```python
from build123d import *

# Parameters (mm, degrees)
MODEL_R             = 1.75
MODEL_R_2           = 2.25
MODEL_R_3           = 15
MODEL_R_4           = 2.75
MODEL_R_5           = 10.5
MODEL_R_6           = 4.25
BOSS_EXTRUDE1_DEPTH = 18


with BuildPart() as part:
    # Model → Boss-Extrude1 (new body)
    with BuildSketch(Plane.XY):
        Polygon((195, 0), (205, 10), (205, 141.83), (195, 151.83), (160.9225, 151.83), (95.411764706, 258.588235294), (54, 300), (16, 300), (0, 284), (0, 90), (10, 80), (65, 80), (75, 70), (75, 10), (85, 0), align=None)
        with Locations((60, 279.7)):
            Circle(MODEL_R, mode=Mode.SUBTRACT)
        with Locations((10, 279.7)):
            Circle(MODEL_R, mode=Mode.SUBTRACT)
        with Locations((10, 224.7)):
            Circle(MODEL_R, mode=Mode.SUBTRACT)
        with Locations((10, 154.7)):
            Circle(MODEL_R, mode=Mode.SUBTRACT)
        with Locations((10, 99.7)):
            Circle(MODEL_R, mode=Mode.SUBTRACT)
        with Locations((60, 99.7)):
            Circle(MODEL_R, mode=Mode.SUBTRACT)
        with Locations((60, 154.7)):
            Circle(MODEL_R, mode=Mode.SUBTRACT)
        with Locations((60, 224.7)):
            Circle(MODEL_R, mode=Mode.SUBTRACT)
        with Locations((10, 252.2)):
            Circle(MODEL_R, mode=Mode.SUBTRACT)
        with Locations((60, 252.2)):
            Circle(MODEL_R, mode=Mode.SUBTRACT)
        with Locations((35, 224.7)):
            Circle(MODEL_R, mode=Mode.SUBTRACT)
        with Locations((10, 189.7)):
            Circle(MODEL_R, mode=Mode.SUBTRACT)
        with Locations((60, 189.7)):
            Circle(MODEL_R, mode=Mode.SUBTRACT)
        with Locations((10, 127.2)):
            Circle(MODEL_R, mode=Mode.SUBTRACT)
        with Locations((60, 127.2)):
            Circle(MODEL_R, mode=Mode.SUBTRACT)
        with Locations((35, 154.7)):
            Circle(MODEL_R, mode=Mode.SUBTRACT)
        with Locations((91.54, 11.5)):
            Circle(MODEL_R_2, mode=Mode.SUBTRACT)
        with Locations((123.86, 11.5)):
            Circle(MODEL_R_2, mode=Mode.SUBTRACT)
        with Locations((156.18, 11.5)):
            Circle(MODEL_R_2, mode=Mode.SUBTRACT)
        with Locations((188.5, 11.5)):
            Circle(MODEL_R_2, mode=Mode.SUBTRACT)
        with Locations((50.5, 205.2)):
            Circle(MODEL_R, mode=Mode.SUBTRACT)
        with Locations((50.5, 174.2)):
            Circle(MODEL_R, mode=Mode.SUBTRACT)
        with Locations((35, 189.7)):
            Circle(MODEL_R_3, mode=Mode.SUBTRACT)
        with Locations((19.5, 174.2)):
            Circle(MODEL_R, mode=Mode.SUBTRACT)
        with Locations((19.5, 205.2)):
            Circle(MODEL_R, mode=Mode.SUBTRACT)
        with Locations((11.45, 213.25)):
            Circle(MODEL_R_4, mode=Mode.SUBTRACT)
        with Locations((58.55, 213.25)):
            Circle(MODEL_R_4, mode=Mode.SUBTRACT)
        with Locations((58.55, 166.15)):
            Circle(MODEL_R_4, mode=Mode.SUBTRACT)
        with Locations((11.45, 166.15)):
            Circle(MODEL_R_4, mode=Mode.SUBTRACT)
        with Locations((35, 111.81)):
            Circle(MODEL_R_5, mode=Mode.SUBTRACT)
        with Locations((35, 267.61)):
            Circle(MODEL_R_5, mode=Mode.SUBTRACT)
        with Locations((89.43, 89.83)):
            Circle(MODEL_R_6, mode=Mode.SUBTRACT)
        with Locations((124.43, 89.83)):
            Circle(MODEL_R_6, mode=Mode.SUBTRACT)
        with Locations((145.88, 135.38)):
            Circle(MODEL_R_4, mode=Mode.SUBTRACT)
        with Locations((192.98, 135.38)):
            Circle(MODEL_R_4, mode=Mode.SUBTRACT)
        with Locations((192.98, 88.28)):
            Circle(MODEL_R_4, mode=Mode.SUBTRACT)
        with Locations((145.88, 88.28)):
            Circle(MODEL_R_4, mode=Mode.SUBTRACT)
        with Locations((169.43, 111.83)):
            Circle(MODEL_R_3, mode=Mode.SUBTRACT)
        with Locations((153.93, 96.33)):
            Circle(MODEL_R, mode=Mode.SUBTRACT)
        with Locations((184.93, 127.33)):
            Circle(MODEL_R, mode=Mode.SUBTRACT)
        with Locations((184.93, 96.33)):
            Circle(MODEL_R, mode=Mode.SUBTRACT)
        with Locations((153.93, 127.33)):
            Circle(MODEL_R, mode=Mode.SUBTRACT)
        with BuildLine():
            Line((89.29, 66.7), (89.29, 62.7))
            ThreePointArc((89.29, 62.7), (91.54, 60.45), (93.79, 62.7))
            Line((93.79, 62.7), (93.79, 66.7))
            ThreePointArc((93.79, 66.7), (91.54, 68.95), (89.29, 66.7))
        make_face(mode=Mode.SUBTRACT)
        with BuildLine():
            Line((121.61, 66.7), (121.61, 62.7))
            ThreePointArc((121.61, 62.7), (123.86, 60.45), (126.11, 62.7))
            Line((126.11, 62.7), (126.11, 66.7))
            ThreePointArc((126.11, 66.7), (123.86, 68.95), (121.61, 66.7))
        make_face(mode=Mode.SUBTRACT)
        with BuildLine():
            Line((153.93, 66.7), (153.93, 62.7))
            ThreePointArc((153.93, 62.7), (156.18, 60.45), (158.43, 62.7))
            Line((158.43, 62.7), (158.43, 66.7))
            ThreePointArc((158.43, 66.7), (156.18, 68.95), (153.93, 66.7))
        make_face(mode=Mode.SUBTRACT)
        with BuildLine():
            Line((186.25, 66.7), (186.25, 62.7))
            ThreePointArc((186.25, 62.7), (188.5, 60.45), (190.75, 62.7))
            Line((190.75, 62.7), (190.75, 66.7))
            ThreePointArc((190.75, 66.7), (188.5, 68.95), (186.25, 66.7))
        make_face(mode=Mode.SUBTRACT)
    extrude(amount=BOSS_EXTRUDE1_DEPTH)


solid = part.part
```
Work out the finished part from the listing and answer in its coordinate system (mm). A direction names the side the tool comes from. Round coordinates to 2 decimals unless told otherwise and drop trailing zeros. Write each loop counter-clockwise with the first axis right and the second up, starting at its lowest first coordinate (ties: lowest second). Pieces come first, ordered by that corner, then holes. Notation, with made-up numbers: (65, 24) - (89, 24) arc R18 ccw to (89, 47) - close; hole circle Ø2 at (27, 22.25). An arc over 180 degrees is marked (long way). Return JSON: item names as keys, results as strings. Group by question number.
Q1. Find the intervals of material crossed by L1, parallel to X at y = 127.33, z = 10.25; L2, parallel to X at y = 99, z = 8; L3, parallel to Y at x = 19.5, z = 1.5, in increasing order.
Q2. The part is cut by section A-A on y = 264. Write down the section's boundary in (x, z), then the cut area to 3 significant figures.
Q3. The part is cut by section B-B on z = 8. Count the separate pieces of the cut face and the enclosed holes in it, then the cut area to 3 significant figures.
Q4. Each of these flat-tipped pins is pushed along its axis until it touches: pin 1 Ø2 at (x, y) = (184.93, 127.33) entering from -Z; pin 2 Ø3 at (x, z) = (23, 14.5) entering from -Y; pin 3 Ø5 at (x, z) = (71.5, 12.5) entering from +Y; pin 4 Ø10 at (y, z) = (189, 14) entering from +X. Where does it stop, or does it pass through?
Q5. The mould has two halves that part along Y. Classify faces 4 (the flat face through (8, 292, 9)), 5 (the cylindrical face through (10.854, 210.565, 8.874)), 6 (the flat face through (80, 5, 9)): released by +Y, released by -Y, zero draft, split by the parting line, or undercut.
Q6. For faces 1 (the flat face through (178, 151.83, 9)), 2 (the flat face through (37, 80, 9)), 3 (the cylindrical face through (194.25, 132.94, 8.87)), determine the directions among +Z, -Z, +X, -X, +Y, -Y from which every point of the face is accessible in a straight line to the end or side of a thin tool.
Solved:
{
 "1": {"L1": "0 to 8.25, 11.75 to 58.25, 61.75 to 152.18, 155.68 to 183.18, 186.68 to 205", "L2": "0 to 8.4, 11.6 to 58.4, 61.6 to 161.66, 177.2 to 205", "L3": "80 to 172.45, 175.95 to 203.45, 206.95 to 300"},
 "2": {"outline": "(0, 0) - (25.14, 0) - (25.14, 18) - (0, 18) - close; (44.86, 0) - (90, 0) - (90, 18) - (44.86, 18) - close", "area": "1,270 mm²"},
 "3": {"separate pieces": "1", "enclosed holes": "46", "area": "38,800 mm²"},
 "4": {"pin 1": "through", "pin 2": "y = 80", "pin 3": "y = 285", "pin 4": "x = 141.18"},
 "5": {"face 4": "released by +Y", "face 5": "undercut", "face 6": "released by -Y"},
 "6": {"face 1": "+Z, -Z, +X, +Y", "face 2": "+Z, -Z, -X, -Y", "face 3": "+Z, -Z"}
}
